The drawing under review shows one solid part. Ordinate dimensions are in mm from its lowest x, y, z. Coordinates: 2 decimals unless noted, no trailing zeros. Order: outer loops, then holes, each group sorted by start corner. A loop starts at its lowest first (then second) coordinate and runs counter-clockwise, first axis right, second up. Notation, with made-up numbers: (5.25, 72.5) - (44.25, 72.5) arc R24 cw to (44.25, 104.5) - close; hole circle Ø4 at (63.5, 41). An arc over 180 degrees is marked (long way). Answer in a Markdown table with one row per item.
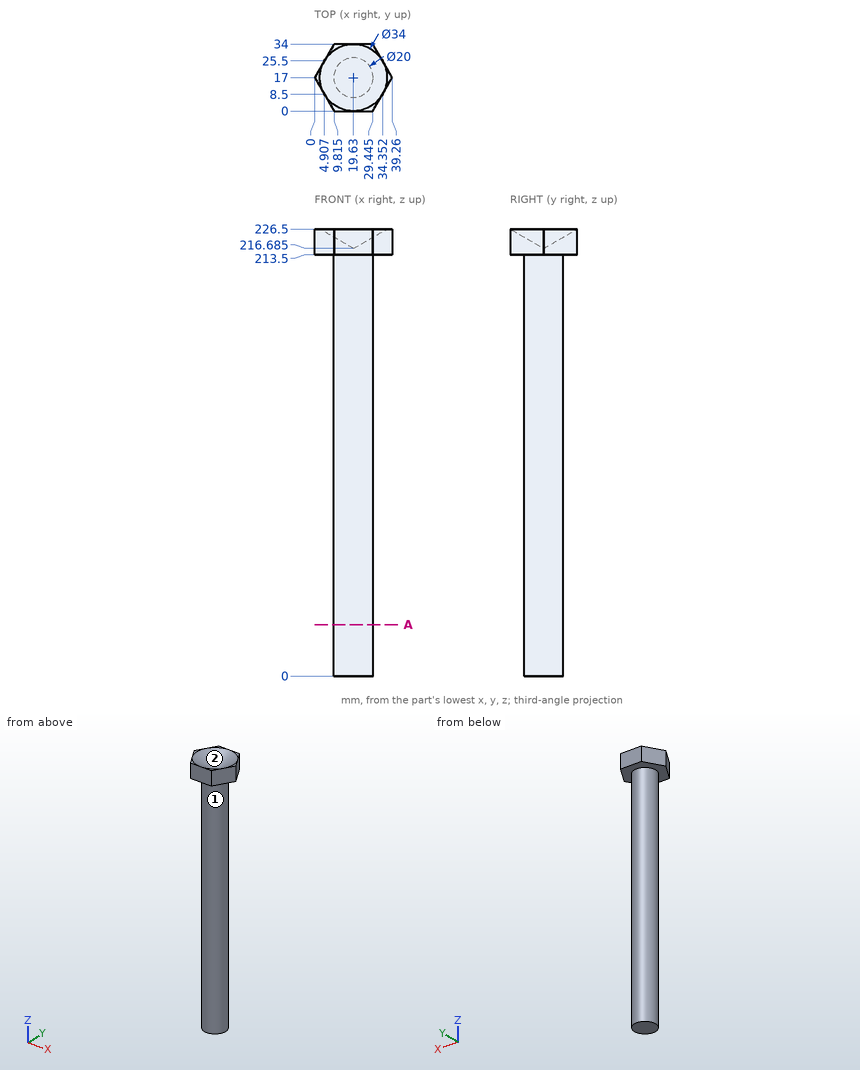
Item 1: Clearance check with flat-ended pins moving along their axes: pin 1 Ø2 at (y, z) = (22, 173.5) entering from -X (1 decimal); pin 2 Ø5 at (x, z) = (28.5, 31) entering from -Y; pin 3 Ø1.5 at (x, z) = (28.5, 139) entering from +Y (1 decimal). State where each tip first meets the part, or that it passes through.
Check values:
| item | result |
|---|---|
| pin 1 | x = 10.5 |
| pin 2 | y = 9.29 |
| pin 3 | y = 22.8 |
Item 2: We need section A-A, the plane z = 26. Write out the cut boundary in (x, y), then the cut area to 3 significant figures.
Check values:
| item | result |
|---|---|
| outline | circle Ø20 at (19.63, 17) |
| area | 314 mm^2 |
Item 3: Mouldability with a two-part tool opening along X and no side actions: class the marked faces 1 and 2 as +X half, -X half, draft (parallel to the pull), parting line (faces both ways), or undercut.
Check values:
| item | result |
|---|---|
| face 1 | parting line |
| face 2 | undercut |
Item 4: To check wall thickness, follow line 1 (X direction, y = 19, z = 97.5); line 2 (Z direction, x = 37, y = 14); line 3 (Y direction, x = 28, z = 15.5) (1 decimal). State the ranges of each line that lie inside material, in increasing order. Write a range as from..to.
Check values:
| item | result |
|---|---|
| line 1 | 9.83..29.43 |
| line 2 | 213.5..226.5 |
| line 3 | 11.5..22.5 |
